Source: CAD feature listing. Evaluate the final solid. Frame: model axes, mm. A direction names the side the tool comes from. Give positions to 0.01 mm unless a question says otherwise; leave off trailing zeros. Put each result on its own line as item: value.
Autodesk Inventor part; units mm, degrees
ref_plane "YZ Plane" through (0, 0, 0) normal (1, 0, 0) x (0, 1, 0)
ref_plane "XZ Plane" through (0, 0, 0) normal (0, 1, 0) x (-1, 0, 0)
ref_plane "XY Plane" through (0, 0, 0) normal (0, 0, 1) x (1, 0, 0)
sketch "Sketch1" plane through (0, 0, 0) normal (0, 1, 0) x (-1, 0, 0)
  line L0 (0, 0) -> (116.2, 0)
  line L1 (116.2, 0) -> (116.2, -252.75)
  line L2 (116.2, -252.75) -> (0, -252.75)
  line L3 (0, -252.75) -> (0, 0)
  dimension "d0" = 116.2
  dimension "d1" = 252.75
extrude "Extrusion1" add sketch "Sketch1" along normal blind 5
sketch "Sketch2" plane through (0, 5, 0) normal (0, 1, 0) x (1, 0, 0)
  line L0 (-143.9049, 8) -> (61.1103, 8) construction
  line L1 (-143.9049, 246.75) -> (56.0412, 246.75) construction
  line L2 (-116.2, 0) -> (0, 0) construction
  line L3 (0, 252.75) -> (-116.2, 252.75) construction
  line L4 (0, 0) -> (0, 252.75) construction
  point P0 (-12, 8)
  point P1 (-43, 8)
  point P2 (-12, 246.75)
  point P3 (-24, 246.75)
  dimension "d4" = 8
  dimension "d5" = 6
  dimension "d6" = 12
  dimension "d7" = 12
  dimension "d8" = 12
  dimension "d9" = 31
hole "Hole1" at (-12, 5, -8) at (-43, 5, -8) at (-12, 5, -246.75) at (-24, 5, -246.75) direction (0, -1, 0) diameter 3.8 end through all
sketch "Sketch3" plane through (0, 5, 0) normal (0, 1, 0) x (1, 0, 0)
  line L0 (-60, 274.5902) -> (-60, -21.6249) construction
  line L1 (0, 0) -> (0, 252.75) construction
  line L2 (0, 252.75) -> (-116.2, 252.75) construction
  line L3 (-116.2, 0) -> (0, 0)
  point P0 (-60, 24)
  point P1 (-60, 12)
  dimension "d17" = 60
  dimension "d19" = 12
  dimension "d27" = 12
hole "Hole2" at (-60, 5, -24) at (-60, 5, -12) direction (0, -1, 0) diameter 3.8 end through all
sketch "Sketch4" plane through (0, 5, 0) normal (0, 1, 0) x (1, 0, 0)
  line L0 (-150.2588, 199) -> (49.1975, 199) construction
  line L1 (0, 252.75) -> (-116.2, 252.75) construction
  line L2 (-97.7, 275.0226) -> (-97.7, 149.5028) construction
  line L3 (-116.2, 252.75) -> (-116.2, 0) construction
  point P0 (0, 0)
  point P1 (-97.7, 211)
  point P2 (-97.7, 223)
  dimension "d28" = 53.75
  dimension "d29" = 18.5
  dimension "d30" = 12
  dimension "d31" = 24
hole "Hole3" at (-97.7, 5, -211) at (-97.7, 5, -223) direction (0, -1, 0) diameter 3.8 end through all
sketch "Sketch6" plane through (0, 5, 0) normal (0, 1, 0) x (1, 0, 0)
  line L0 (-135.4427, 230.25) -> (59.7258, 230.25) construction
  line L1 (0, 252.75) -> (-116.2, 252.75) construction
  line L2 (-116.2, 252.75) -> (-116.2, 0) construction
  point P0 (0, 0)
  point P1 (-99.5, 230.25)
  point P2 (-49.5, 230.25)
  dimension "d50" = 22.5
  dimension "d51" = 16.7
  dimension "d52" = 66.7
hole "Hole5" at (-99.5, 5, -230.25) at (-49.5, 5, -230.25) direction (0, -1, 0) diameter 3.8 end through all
sketch "Sketch7" plane through (0, 5, 0) normal (0, 1, 0) x (1, 0, 0)
  line L0 (0, 252.75) -> (-116.2, 252.75)
  line L1 (-116.2, 252.75) -> (-116.2, 0)
  circle A0 centre (-66.278, 89.237) radius 12
  line L2 (-66.278, 89.237) -> (-96.1481, 98.9825)
  point P0 (0, 0)
  point P1 (-77.6862, 92.9591)
  dimension "d64" = 24
  dimension "d60" = 163.513
  dimension "d61" = 49.922
  dimension "d73" = 71.93
hole "Hole6" at (-66.278, 5, -89.237) at (-77.6862, 5, -92.9591) direction (0, -1, 0) diameter 3.8 end through all
sketch "Sketch8" plane through (0, 5, 0) normal (0, 1, 0) x (1, 0, 0)
  line L0 (-136.1371, 23.25) -> (33.8661, 23.25) construction
  line L1 (-116.2, 0) -> (0, 0) construction
  line L2 (-116.2, 252.75) -> (-116.2, 0) construction
  point P0 (-100.2, 23.25)
  point P1 (-42.7, 23.25)
  dimension "d74" = 23.25
  dimension "d75" = 16
  dimension "d76" = 73.5
hole "Hole7" at (-100.2, 5, -23.25) at (-42.7, 5, -23.25) direction (0, -1, 0) diameter 3.8 end through all
sketch "Sketch9" plane through (0, 5, 0) normal (0, 1, 0) x (1, 0, 0)
  line L0 (-125.6401, 227.25) -> (33.4538, 227.25) construction
  line L1 (0, 252.75) -> (-116.2, 252.75)
  line L2 (0, 0) -> (0, 252.75)
  line L3 (-167.8122, 196.25) -> (35.3783, 196.25) construction
  line L4 (-116.2, 252.75) -> (-116.2, 0)
  point P0 (-24, 227.25)
  point P1 (-84, 227.25)
  point P2 (-84, 196.25)
  point P3 (-46, 196.25)
  point P4 (-109.5, 226.25)
  dimension "d84" = 25.5
  dimension "d85" = 24
  dimension "d86" = 84
  dimension "d94" = 56.5
  dimension "d95" = 84
  dimension "d96" = 46
  dimension "d97" = 26.5
  dimension "d98" = 6.7
hole "Hole8" at (-24, 5, -227.25) at (-84, 5, -227.25) at (-84, 5, -196.25) at (-46, 5, -196.25) at (-109.5, 5, -226.25) direction (0, -1, 0) diameter 3.8 end through all
sketch "Sketch10" plane through (0, 5, 0) normal (0, 1, 0) x (1, 0, 0)
  line L0 (-109.7, 267.6136) -> (-109.7, -16.6151) construction
  line L1 (-116.2, 252.75) -> (-116.2, 0) construction
  line L2 (0, 252.75) -> (-116.2, 252.75)
  point P0 (0, 0)
  point P1 (-109.7, 234)
  point P2 (-109.7, 22.25)
  dimension "d99" = 6.5
  dimension "d100" = 18.75
  dimension "d101" = 211.75
hole "Hole9" at (-109.7, 5, -234) at (-109.7, 5, -22.25) direction (0, -1, 0) diameter 3.8 end through all
sketch "Sketch11" plane through (0, 5, 0) normal (0, 1, 0) x (1, 0, 0)
  line L0 (-96.7, 85.8638) -> (-96.7, -44.5279) construction
  line L1 (-141.7957, 6) -> (-51.6043, 6) construction
  line L2 (-116.2, 0) -> (0, 0)
  line L3 (-116.2, 252.75) -> (-116.2, 0)
  point P0 (-96.7, 45)
  point P1 (-96.7, 84)
  point P2 (-96.7, 6)
  dimension "d109" = 6
  dimension "d110" = 19.5
  dimension "d111" = 39
  dimension "d112" = 39
hole "Hole10" at (-96.7, 5, -45) at (-96.7, 5, -84) at (-96.7, 5, -6) direction (0, -1, 0) diameter 3.8 end through all
sketch "Sketch12" plane through (0, 5, 0) normal (0, 1, 0) x (1, 0, 0)
  line L0 (-148.2315, 164.75) -> (24.3981, 164.75) construction
  line L1 (0, 252.75) -> (-116.2, 252.75)
  line L2 (0, 0) -> (0, 252.75)
  point P0 (-20, 164.75)
  point P1 (-85, 164.75)
  dimension "d120" = 88
  dimension "d121" = 20
  dimension "d122" = 85
hole "Hole11" at (-20, 5, -164.75) at (-85, 5, -164.75) direction (0, -1, 0) diameter 3.8 end through all
sketch "Sketch13" plane through (0, 5, 0) normal (0, 1, 0) x (1, 0, 0)
  line L0 (-159.8751, 114) -> (39.6093, 114) construction
  line L1 (-116.2, 0) -> (0, 0) construction
  line L2 (-96.2, 94) -> (-136.2, 94)
  line L3 (-136.2, 94) -> (-136.2, 134)
  line L4 (-136.2, 134) -> (-96.2, 134)
  line L5 (-96.2, 134) -> (-96.2, 94)
  line L6 (-116.2, 252.75) -> (-116.2, 0) construction
  line L7 (-96.2, 94) -> (-136.2, 134) construction
  line L8 (-136.2, 94) -> (-96.2, 134) construction
  point P0 (-116.2, 114)
  dimension "d130" = 114
  dimension "d131" = 40
  dimension "d132" = 40
extrude "Extrusion2" cut sketch "Sketch13" against normal through all
fillet "Fillet1" radius 4 4 edges at (-116.2, 2.5, -134) (-116.2, 2.5, -94) (-96.2, 2.5, -94) (-96.2, 2.5, -134)
fillet "Fillet2" radius 2 1 edges at (-116.2, 2.5, -252.75)
properties part number "Internal Vert Divider"
1) Material intervals for line 1 along Z through (x, y) = (-12, 3.4); line 2 along X through (y, z) = (2.9, -8); line 3 along X through (y, z) = (2.55, -223), sorted ascending. Write a range as [from, to].
Check result:
line 1: [-252.75, -248.65], [-244.85, -9.9], [-6.1, 0]
line 2: [-116.2, -44.9], [-41.1, -13.9], [-10.1, 0]
line 3: [-116.2, -99.6], [-95.8, 0]
2) Section query A-A, the plane y = 3.45. State how many separate pieces and enclosed holes the cut face has, plus the area to 3 significant figures.
Check result:
separate pieces: 1
enclosed holes: 26
area: 28,300 mm²
3) Mould query, pull axis Z, two halves, no side actions, for faces 3 (the flat face through (-106, 3, -94)), 4 (the flat face through (-116.2, 2, -44)), 5 (the flat face through (-58, 2, -252.75)). Classes: pulls with the +Z half, pulls with the -Z half, needs draft (parallel to the pull), parting line crosses it, or undercut.
Check result:
face 3: undercut
face 4: needs draft
face 5: pulls with the -Z half
4) Pin query (flat end, axial travel): P1, Ø1.5, axis at y = 4.5, z = -50, coming from the +X side; P2, Ø3.5, axis at x = -60, z = -12, coming from the -Y side. Return the tip coordinate at first contact, or that it passes through.
Check result:
P1: x = 0
P2: through
5) Access query for faces 1 (the flat face through (-96.2, 3, -114)), 2 (the flat face through (-116.2, 2, -194)). Directions: +Z, -Z, +X, -X, +Y, -Y. A direction counts if a zero-diameter tool reaches every point of the face in a straight line with its end or side. Return the directions, or none.
Check result:
face 1: -X, +Y, -Y
face 2: +Z, -Z, -X, +Y, -Y
